```python
from build123d import *

# Parameters (mm, degrees)
SKIZZE1_W                       = 300
SKIZZE1_H                       = 90.0015
AUFSATZ_LINEAR_AUSTRAGEN1_DEPTH = 3
DURCHGANGSLOCH_F_R_M61_D        = 6.6
SKIZZE4_W                       = 8
SKIZZE4_H                       = 18
SCHNITT_LINEAR_AUSTRAGEN1_DEPTH = 10
SCHNITT_LINEAR_AUSTRAGEN2_DEPTH = 10


with BuildPart() as part:
    # Skizze1 → Aufsatz-Linear austragen1 (new body)
    with BuildSketch(Plane.XY):
        with Locations((-150, -29.999999991)):
            Rectangle(SKIZZE1_W, SKIZZE1_H)
    extrude(amount=AUFSATZ_LINEAR_AUSTRAGEN1_DEPTH)

    # Durchgangsloch für M61 (through all)
    with Locations(Plane.XY.offset(3)):
        with Locations((-15, 0.000750009), (-15, -60.000749991), (-285, -60.000749991), (-285, 0.000750009)):
            Hole(DURCHGANGSLOCH_F_R_M61_D / 2)

    # Skizze4 → Schnitt-Linear austragen1 (cut)
    with BuildSketch(Plane.XY.offset(3)):
        with Locations((-269, -28.999249991)):
            Rectangle(SKIZZE4_W, SKIZZE4_H)
        with Locations((-249, -28.999249991)):
            Rectangle(SKIZZE4_W, SKIZZE4_H)
        with Locations((-229, -28.999249991)):
            Rectangle(SKIZZE4_W, SKIZZE4_H)
    extrude(amount=-SCHNITT_LINEAR_AUSTRAGEN1_DEPTH, mode=Mode.SUBTRACT)

    # Skizze5 → Schnitt-Linear austragen2 (cut)
    with BuildSketch(Plane.XY.offset(3)):
        with BuildLine():
            Line((-34.255252171, -23.380072644), (-39.238223172, -23.380072644))
            ThreePointArc((-39.238223172, -23.380072644), (-41.846737672, -27.830072644), (-39.238223172, -32.280072644))
            Line((-39.238223172, -32.280072644), (-34.255252171, -32.280072644))
            ThreePointArc((-34.255252171, -32.280072644), (-31.646737672, -27.830072644), (-34.255252171, -23.380072644))
        make_face()
    extrude(amount=-SCHNITT_LINEAR_AUSTRAGEN2_DEPTH, mode=Mode.SUBTRACT)


solid = part.part
```
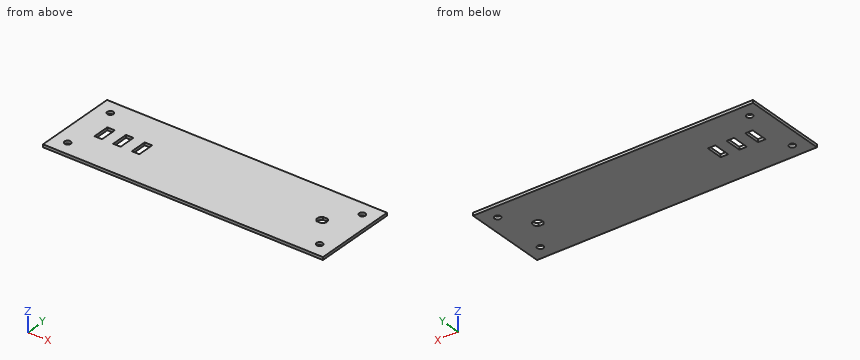
Design review of the part built by this model. Coordinates are the model's own, in mm. Round coordinates to 2 decimals unless told otherwise and drop trailing zeros. Write each loop counter-clockwise with the first axis right and the second up, starting at its lowest first coordinate (ties: lowest second). Pieces come first, ordered by that corner, then holes.
Item 1: We need section B-B on z = 2.15. State how many separate pieces and enclosed holes the cut face has, and give its area (3 significant figures).
Item 2: For probe 1 along Y at (x, z) = (-285, 1.5); probe 2 along X at (y, z) = (-22, 0.35); probe 3 along X at (y, z) = (-31.5, 0.25), list the stretches that pass through material, from the lowest coordinate up.
Item 3: We need section A-A on x = -15. Write out the cut boundary in (y, z), and give its area (3 significant figures).
Returned:
1. separate pieces: 1
1. enclosed holes: 8
1. area: 26,400 mm2
2. probe 1: y = -75 to -63.3, -56.7 to -3.3, 3.3 to 15
2. probe 2: x = -300 to -273, -265 to -253, -245 to -233, -225 to 0
2. probe 3: x = -300 to -273, -265 to -253, -245 to -233, -225 to -40.29, -33.21 to 0
3. outline: (-75, 0) - (-63.3, 0) - (-63.3, 3) - (-75, 3) - close; (-56.7, 0) - (-3.3, 0) - (-3.3, 3) - (-56.7, 3) - close; (3.3, 0) - (15, 0) - (15, 3) - (3.3, 3) - close
3. area: 230 mm2
